from build123d import *

# Parameters (mm, degrees)
SCHIZZO1_W                   = 99
SCHIZZO1_H                   = 51
ESTRUSIONE_ESTRUSIONE1_DEPTH = 44
SCHIZZO2_W                   = 55
SCHIZZO2_H                   = 51
TAGLIO_ESTRUSIONE1_DEPTH     = 6
SCHIZZO3_W                   = 41
SCHIZZO3_H                   = 18
TAGLIO_ESTRUSIONE2_DEPTH     = 3
SCHIZZO4_W                   = 9
SCHIZZO4_H                   = 51
TAGLIO_ESTRUSIONE3_DEPTH     = 6
SCHIZZO5_W                   = 41
SCHIZZO5_H                   = 19
TAGLIO_ESTRUSIONE4_DEPTH     = 118.669027361
SCHIZZO6_W                   = 13
SCHIZZO6_H                   = 25
TAGLIO_ESTRUSIONE5_DEPTH     = 120.741387999
SCHIZZO7_W                   = 67
SCHIZZO7_H                   = 19
ESTRUSIONE_ESTRUSIONE2_DEPTH = 10
TAGLIO_ESTRUSIONE6_DEPTH     = 108.670794555
RACCORDO1_R                  = 6


with BuildPart() as part:
    # Schizzo1 → Estrusione-Estrusione1 (new body)
    with BuildSketch(Plane(origin=(0, 0, 0), x_dir=(1, 0, 0), z_dir=(0, 1, 0))):
        with Locations((-49.5, 25.5)):
            Rectangle(SCHIZZO1_W, SCHIZZO1_H)
    extrude(amount=ESTRUSIONE_ESTRUSIONE1_DEPTH)

    # Schizzo2 → Taglio-Estrusione1 (cut)
    with BuildSketch(Plane(origin=(0, 44, 0), x_dir=(1, 0, 0), z_dir=(0, 1, 0))):
        with Locations((-27.5, 25.5)):
            Rectangle(SCHIZZO2_W, SCHIZZO2_H)
    extrude(amount=-TAGLIO_ESTRUSIONE1_DEPTH, mode=Mode.SUBTRACT)

    # Schizzo3 → Taglio-Estrusione2 (cut)
    with BuildSketch(Plane(origin=(0, 44, 0), x_dir=(1, 0, 0), z_dir=(0, 1, 0))):
        with Locations((-78.5, 15)):
            Rectangle(SCHIZZO3_W, SCHIZZO3_H)
    extrude(amount=-TAGLIO_ESTRUSIONE2_DEPTH, mode=Mode.SUBTRACT)

    # Schizzo4 → Taglio-Estrusione3 (cut)
    with BuildSketch(Plane(origin=(0, 44, 0), x_dir=(1, 0, 0), z_dir=(0, 1, 0))):
        with Locations((-77.5, 25.5)):
            Rectangle(SCHIZZO4_W, SCHIZZO4_H)
    extrude(amount=-TAGLIO_ESTRUSIONE3_DEPTH, mode=Mode.SUBTRACT)

    # Schizzo5 → Taglio-Estrusione4 (cut, through all)
    with BuildSketch(Plane(origin=(0, 38, 0), x_dir=(1, 0, 0), z_dir=(0, 1, 0))):
        with Locations((-20.5, 25.5)):
            Rectangle(SCHIZZO5_W, SCHIZZO5_H)
    extrude(amount=-TAGLIO_ESTRUSIONE4_DEPTH, mode=Mode.SUBTRACT)

    # Schizzo6 → Taglio-Estrusione5 (cut, through all)
    with BuildSketch(Plane.XY):
        with Locations((-92.5, 12.5)):
            Rectangle(SCHIZZO6_W, SCHIZZO6_H)
    extrude(amount=-TAGLIO_ESTRUSIONE5_DEPTH, mode=Mode.SUBTRACT)

    # Schizzo7 → Estrusione-Estrusione2 (add)
    with BuildSketch(Plane.XY):
        with Locations((-48.5, 22.5)):
            Rectangle(SCHIZZO7_W, SCHIZZO7_H)
    extrude(amount=ESTRUSIONE_ESTRUSIONE2_DEPTH)

    # Schizzo8 → Taglio-Estrusione6 (cut, through all)
    with BuildSketch(Plane(origin=(-15, 0, 0), x_dir=(0, 0, -1), z_dir=(1, 0, 0))):
        Polygon((0, 32), (-10, 15), (-10, 32), align=None)
    extrude(amount=-TAGLIO_ESTRUSIONE6_DEPTH, mode=Mode.SUBTRACT)

    # Raccordo1
    raccordo1_edges = [part.edges().sort_by_distance(p)[0] for p in [
        (-55, 38, -25.5),
    ]]
    fillet(raccordo1_edges, radius=RACCORDO1_R - 0.0001)  # a hair under: the kernel refuses the full size


solid = part.part
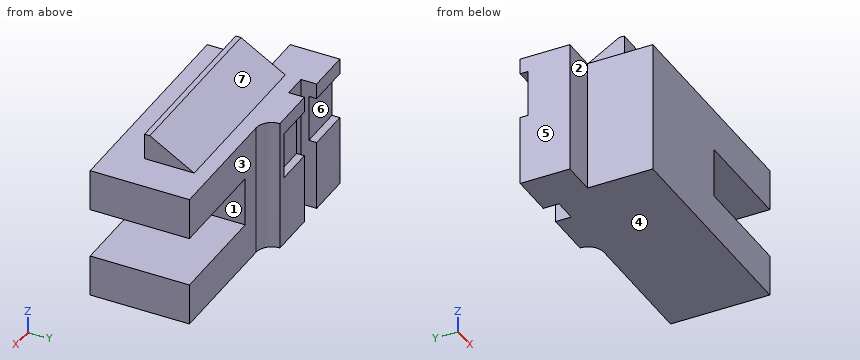
Design review of the part built by this model. Coordinates are the model's own, in mm. Face numbers are marked on the shaded views. A direction names the side the tool comes from. Round coordinates to 2 decimals unless told otherwise and drop trailing zeros. Write each loop counter-clockwise with the first axis right and the second up, starting at its lowest first coordinate (ties: lowest second). Pieces come first, ordered by that corner, then holes.
Item 1: Consider section D-D on x = -60.5. Give the boundary of the cut face in (y, z), and give its area (4 significant figures).
Item 2: Wall thickness on L1, parallel to Z at x = -30, y = 4; L2, parallel to Y at x = -86.5, z = -14.5; L3, parallel to X at y = 17, z = -9: over which ranges is each line inside the solid? List them lowest first.
Item 3: Consider section A-A on x = -30.5. Give the boundary of the cut face in (y, z).
Item 4: Draft analysis for pull direction Z (two halves, no side actions). For the marked faces 4, 5, 6 and 7, state which applies: released by +Z, released by -Z, zero draft, split by the parting line, or undercut.
Item 5: For pin 1 Ø5 at (x, z) = (-59.5, 5) entering from -Y; pin 2 Ø1.5 at (x, y) = (-63.5, 42) entering from +Z; pin 3 Ø5 at (y, z) = (41, -21.5) entering from +X, all flat-tipped, find the tip position at first contact; note any pin that passes through.
Item 6: For the marked faces 1, 2 and 3, list the 3-axis set-ups (+Z, -Z, +X, -X, +Y, -Y) from which the entire face can be reached by the end or side of a thin tool; tool diameter is ignored.
Item 7: Consider section B-B on y = 40. Give the boundary of the cut face in (x, z).
Check values:
1. outline: (0, -51) - (44, -51) - (44, -24) - (41, -24) - (41, -6) - (44, -6) - (44, 0) - (32, 0) - (15, 10) - (13, 10) - (13, 0) - (0, 0) - close
1. area: 2,295 mm2
2. L1: z = -51 to -35, -16 to 0
2. L2: y = 25 to 41
2. L3: x = -86 to 0
3. outline: (0, -51) - (38, -51) - (38, -35) - (0, -35) - close; (0, -16) - (38, -16) - (38, 0) - (32, 0) - (15, 10) - (13, 10) - (13, 0) - (0, 0) - close
4. face 4: released by -Z
4. face 5: zero draft
4. face 6: undercut
4. face 7: released by +Z
5. pin 1: stops at y = 13
5. pin 2: stops at z = 0
5. pin 3: stops at x = -51.4
6. face 1: +X, +Y, -Y
6. face 2: +Z, -Z, -X, -Y
6. face 3: +Z, -Z, +X, +Y
7. outline: (-99, -51) - (-82, -51) - (-82, 0) - (-99, 0) - close; (-73, -51) - (-53.47, -51) - (-53.47, 0) - (-73, 0) - close
